Geometry check sheet. Reference: drawing and pictorial views, mm from the part's lowest x, y, z. A direction names the side the tool comes from. Coordinates: 2 decimals unless noted, no trailing zeros. Loops run counter-clockwise (first coordinate to the right, second up) from the corner with the lowest first, then second, coordinate; pieces in that order, holes last.
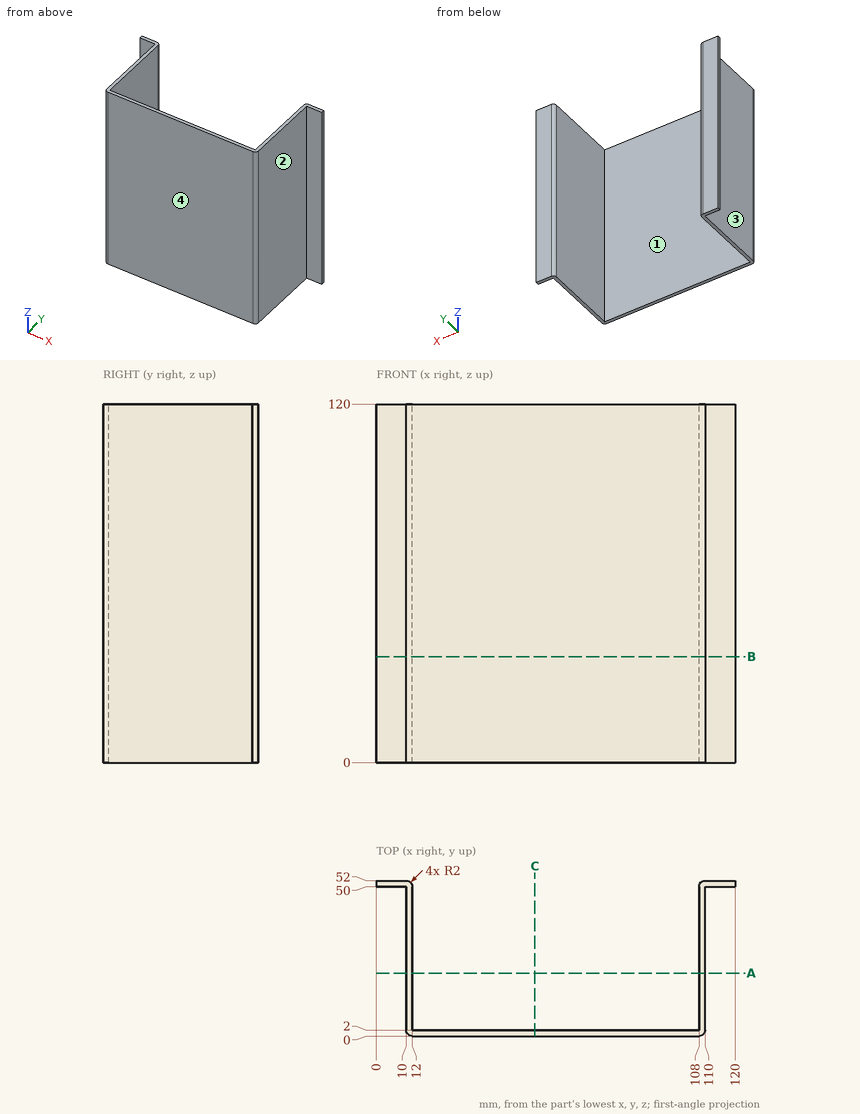
1) Section check A-A on y = 21. Record the cut outline in (x, z).
Data:
outline: (10, 0) - (12, 0) - (12, 120) - (10, 120) - close; (108, 0) - (110, 0) - (110, 120) - (108, 120) - close
2) Section check B-B on z = 35.5. Record the cut outline in (x, y).
Data:
outline: (0, 50) - (10, 50) - (10, 2) arc R2 ccw to (12, 0) - (108, 0) arc R2 ccw to (110, 2) - (110, 50) - (120, 50) - (120, 52) - (110, 52) arc R2 ccw to (108, 50) - (108, 2) - (12, 2) - (12, 50) arc R2 ccw to (10, 52) - (0, 52) - close
3) Section check C-C on x = 53. Record the cut outline in (y, z).
Data:
outline: (0, 0) - (2, 0) - (2, 120) - (0, 120) - close
4) Access from +Z, -Z, +X, -X, +Y, -Y to the whole of each face (thin tool, end or side, straight path). Record for the marked faces 1, 2, 3 and 4.
Data:
face 1: +Z, -Z, +Y
face 2: +Z, -Z, +X, -Y
face 3: +Z, -Z, -X, -Y
face 4: +Z, -Z, +X, -X, -Y
5) Depth check by flat-ended pin: pin 1 (8 mm diameter, centred on x = 59.5, z = 30.5, fed in from +Y); pin 2 (8 mm diameter, centred on x = 3, z = 48.5, fed in from -Y); pin 3 (2 mm diameter, centred on y = 26, z = 39, fed in from +X); pin 4 (6 mm diameter, centred on x = 104, y = 23, fed in from +Z). Enter the tip coordinate at first touch or a pass-through.
Data:
pin 1: stops at y = 2
pin 2: stops at y = 50
pin 3: stops at x = 110
pin 4: passes through
6) Material ranges on probe 1 along X at (y, z) = (11, 102); probe 2 along Y at (x, z) = (57, 56.5); probe 3 along Y at (x, z) = (8, 90.5), recorded low to high.
Data:
probe 1: x = 10 to 12, 108 to 110
probe 2: y = 0 to 2
probe 3: y = 50 to 52
